Verification items for the finished model (mm, model axes). A direction names the side the tool comes from. Round coordinates to 2 decimals unless told otherwise and drop trailing zeros. Write each loop counter-clockwise with the first axis right and the second up, starting at its lowest first coordinate (ties: lowest second). Pieces come first, ordered by that corner, then holes.
from build123d import *

# Parameters (mm, degrees)
F0_R          = 100
F1_DEPTH      = 5
F1_DEPTH_BACK = 25
F2_R          = 100
F2_R_2        = 95
F2_R_3        = 87.5
F2_R_4        = 82.5
F2_R_5        = 75
F2_R_6        = 70
F2_R_7        = 62.5
F2_R_8        = 57.5
F2_R_9        = 50
F2_R_10       = 45
F2_R_11       = 37.5
F2_R_12       = 32.5
F2_R_13       = 25
F2_R_14       = 20
F2_R_15       = 12.5
F2_R_16       = 7.5
F3_DEPTH      = 15
F4_R          = 31.65685
F5_DEPTH      = 5


with BuildPart() as f1:
    # F0 (on Top) → F1 (new body, two sides)
    with BuildSketch(Plane.XY) as f1_sk:
        Circle(F0_R)
    extrude(amount=F1_DEPTH)
    extrude(f1_sk.sketch, amount=-F1_DEPTH_BACK)

    # F2 (on face) → F3 (join)
    with BuildSketch(Plane.XY.offset(5)):
        Circle(F2_R)
        Circle(F2_R_2, mode=Mode.SUBTRACT)
        Circle(F2_R_3)
        Circle(F2_R_4, mode=Mode.SUBTRACT)
        Circle(F2_R_5)
        Circle(F2_R_6, mode=Mode.SUBTRACT)
        Circle(F2_R_7)
        Circle(F2_R_8, mode=Mode.SUBTRACT)
        Circle(F2_R_9)
        Circle(F2_R_10, mode=Mode.SUBTRACT)
        Circle(F2_R_11)
        Circle(F2_R_12, mode=Mode.SUBTRACT)
        Circle(F2_R_13)
        Circle(F2_R_14, mode=Mode.SUBTRACT)
        Circle(F2_R_15)
        Circle(F2_R_16, mode=Mode.SUBTRACT)
    extrude(amount=F3_DEPTH)

    # F4 (on face) → F5 (join)
    with BuildSketch(Plane(origin=(0, 0, -25), x_dir=(1, 0, 0), z_dir=(0, 0, -1))):
        Circle(F4_R)
    extrude(amount=F5_DEPTH)


solid = f1.part
Q1. Tool access check on faces 1 (the flat face through (-24, 24, -25)), 2 (the cylindrical face through (-7.493, 0.33, 12.395)), 3 (the flat face through (0, -8, 20)). Record the directions out of +Z, -Z, +X, -X, +Y, -Y that give a thin tool (end or side, any length) a straight path to the whole face; none if there is none.
Recorded:
face 1: -Z
face 2: +Z
face 3: +Z, +X, -X, +Y, -Y
Q2. Depth check by flat-ended pin: P1, Ø3, axis at y = -38, z = -24, coming from the -X side; P2, Ø4, axis at y = -51.5, z = -9.5, coming from the -X side; P3, Ø12, axis at x = 36, z = -20, coming from the -Y side. Enter the tip coordinate at first touch or a pass-through.
Recorded:
P1: stops at x = -93.1
P2: stops at x = -86.89
P3: stops at y = -95.39
Q3. Sectioned sample at A-A (z = -14). Enter the section's corners in (x, y), plus the area to 3 significant figures.
Recorded:
outline: circle Ø200 at (0, 0)
area: 31,400 mm2
Q4. Release check for a two-part mould opening along X. For faces 4 (the flat face through (88, -37, 20)), 5 (the flat face through (-26.3, 57.4, 5)) record: released by +X, released by -X, zero draft, split by the parting line, or undercut.
Recorded:
face 4: zero draft
face 5: undercut
Q5. Sectioned sample at B-B (x = -66.5). Enter the section's corners in (y, z).
Recorded:
outline: (-74.68, -25) - (74.68, -25) - (74.68, 20) - (67.84, 20) - (67.84, 5) - (56.87, 5) - (56.87, 20) - (48.83, 20) - (48.83, 5) - (34.68, 5) - (34.68, 20) - (21.86, 20) - (21.86, 5) - (-21.86, 5) - (-21.86, 20) - (-34.68, 20) - (-34.68, 5) - (-48.83, 5) - (-48.83, 20) - (-56.87, 20) - (-56.87, 5) - (-67.84, 5) - (-67.84, 20) - (-74.68, 20) - close
Q6. Material ranges on line 1 along Z through (x, y) = (27, -3.5); line 2 along Z through (x, y) = (2.5, -55); line 3 along Y through (x, z) = (-13, 1), recorded low to high.
Recorded:
line 1: z = -30 to 5
line 2: z = -25 to 5
line 3: y = -99.15 to 99.15
